Design review of the part built by this model. Coordinates are the model's own, in mm. Coordinates: 2 decimals unless noted, no trailing zeros. Order: outer loops, then holes, each group sorted by start corner. A loop starts at its lowest first (then second) coordinate and runs counter-clockwise, first axis right, second up. Notation, with made-up numbers: M 81,8.5 L 92,8.5 A17 cw 92,33.5 Z; hole C -40,9 d3. An arc over 180 degrees is marked long. Answer as a JSON object with one key per item and string values.
from build123d import *

# Parameters (mm, degrees)
F1_DEPTH    = 5.08
F2_T1_DEPTH = 107.0884939123
F3_SIZE     = 5.07999


# Not quite as in the source:
# - a fillet or chamfer that OpenCascade refuses, or shapes differently, is made with other operations: its cross-section is extruded or revolved along the edge and cut away or added
# - a fillet or chamfer is up to 0.001 mm smaller than in the source, because OpenCascade refuses the exact size


with BuildPart() as f1:
    # F0 (on Top) → F1 (new body)
    with BuildSketch(Plane.XY):
        Polygon((-52.3975975811, 62.6697838306), (0, 0), (0, 36.2825095654), (-52.3975975811, 79.6330347657), align=None)
    extrude(amount=F1_DEPTH)

    # F2: fillet of radius 5.08 on 2 edges, made by hand

    # F2_s2 → F2_t1 (cut)
    with BuildSketch(Plane(origin=(-60.5437814243, 72.412970619, 0), x_dir=(0, 0, 1), z_dir=(0.6414317987, -0.7671800621, 0))):
        with BuildLine():
            ThreePointArc((0, 0), (3.5921024484, -1.4878975516), (5.08, -5.08))
            Line((5.08, -5.08), (5.08, 0))
            Line((5.08, 0), (0, 0))
        make_face()
        with BuildLine():
            ThreePointArc((5.08, 0), (1.4878975516, -1.4878975516), (0, -5.08))
            Line((0, -5.08), (0, 0))
            Line((0, 0), (5.08, 0))
        make_face()
    extrude(amount=F2_T1_DEPTH, mode=Mode.SUBTRACT)

    # F3 (size 5.08 in the source; OpenCascade refuses exactly that, so slightly less here)
    f3_edges = [f1.edges().sort_by_distance(p)[0] for p in [
        (-26.198799, 57.957772, 5.08),
    ]]
    chamfer(f3_edges, length=F3_SIZE)


solid = f1.part
1) Insertion check: pin 1 Ø3 at (y, z) = (39.5, 3.5) entering from +X. The pin has a flat end and moves straight along its axis. Give the tip position at first contact, or say it passes through.
Taken from the geometry:
{"pin 1": "stops at x = -6.41"}
2) To check wall thickness, follow L1, parallel to Y at x = -45.5, z = 3; L2, parallel to Y at x = -29.5, z = 3.7; L3, parallel to X at y = 6.5, z = 3.55. State the ranges of each line that lie inside material, in increasing order.
Taken from the geometry:
{"L1": "y = 55.95 to 70.03", "L2": "y = 37.78 to 55.89", "L3": "x = -3.55 to 0"}
3) Add section A-A (z = 1.55). State the section outline as (x, y) points, and give its area (3 significant figures).
Taken from the geometry:
{"outline": "M -52.4,64.89 L 0,2.22 L 0,34.27 L -52.4,77.62 Z", "area": "1,170 mm2"}
